Geometry: final body of the model. Coordinates: model frame, mm. A direction names the side the tool comes from. Coordinates: 2 decimals unless noted, no trailing zeros. Write each loop counter-clockwise with the first axis right and the second up, starting at its lowest first coordinate (ties: lowest second). Pieces come first, ordered by that corner, then holes.
Autodesk Inventor part; units mm, degrees
ref_plane "YZ Plane" through (0, 0, 0) normal (1, 0, 0) x (0, 1, 0)
ref_plane "XZ Plane" through (0, 0, 0) normal (0, 1, 0) x (-1, 0, 0)
ref_plane "XY Plane" through (0, 0, 0) normal (0, 0, 1) x (1, 0, 0)
sketch "Szkic1" plane through (0, 0, 0) normal (0, 0, 1) x (1, 0, 0)
  circle A0 centre (0, 0) radius 90
  circle A1 centre (0, 0) radius 90
  circle A2 centre (0, 0) radius 95
  point P0 (0, 0)
  dimension "d0" = 190
extrude "Wyciągnięcie proste1" add sketch "Szkic1" against normal blind 10
ref_plane "Płaszczyzna konstrukcyjna1" through (0, 0, 0) normal (0, 0, 1) x (1, 0, 0)
sketch "Szkic2" plane through (0, 0, 0) normal (0, 0, 1) x (1, 0, 0)
  circle A0 centre (0, 0) radius 95
  circle A1 centre (0, 0) radius 20
  dimension "d3" = 40
extrude "Wyciągnięcie proste2" add sketch "Szkic2" along normal blind 10
fillet "Zaokrąglenie1" radius 10 1 edges at (-95, 0, 10)
chamfer "Faza1" distance 2 angle 45 1 edges at (-95, 0, -10)
chamfer "Faza2" distance 2 angle 45 2 edges at (-20, 0, 0) (-20, 0, 10)
properties part number "dekieltop" material "PCW, nieplastyfikowany"
Item 1: Section A-A, the plane x = 0. Output: boundary loops of the cut face in (y, z).
Derived:
outline: (-95, -8) - (-93, -10) - (-90, -10) - (-90, 0) - (-22, 0) - (-20, 2) - (-20, 8) - (-22, 10) - (-85, 10) arc R10 ccw to (-95, 0) - close; (20, 2) - (22, 0) - (90, 0) - (90, -10) - (93, -10) - (95, -8) - (95, 0) arc R10 ccw to (85, 10) - (22, 10) - (20, 8) - close
Item 2: Set-up query: faces 1 (the flat face through (19, -19, 0)), 2 (the flat face through (-49, 76, -10)). Return all of +Z, -Z, +X, -X, +Y, -Y with unobstructed straight access to the full face (end or side cutting, diameter ignored); none if empty.
Derived:
face 1: -Z
face 2: -Z, +X, -X, +Y, -Y
Item 3: Pin query (flat end, axial travel): pin 1 (1 mm diameter, centred on y = 51, z = -3.5, fed in from +X); pin 2 (3 mm diameter, centred on x = -35.5, z = -6.5, fed in from +Y); pin 3 (1.5 mm diameter, centred on y = -12.5, z = -1.5, fed in from -X); pin 4 (24 mm diameter, centred on x = 0, y = 0, fed in from +Z). Return the tip coordinate at first contact, or that it passes through.
Derived:
pin 1: stops at x = 80.47
pin 2: stops at y = 88.71
pin 3: stops at x = -94.27
pin 4: passes through
Item 4: Material intervals for probe 1 along Y at (x, z) = (0, -7); probe 2 along Z at (x, y) = (59.5, -7.5); probe 3 along X at (y, z) = (-4.5, 8), sorted ascending.
Derived:
probe 1: y = -95 to -90, 90 to 95
probe 2: z = 0 to 10
probe 3: x = -90.89 to -19.49, 19.49 to 90.89
Item 5: Pull-direction query (Y, two-part tool) for faces 3 (the conical face through (88.825, 27.972, -9.875)), 4 (the conical face through (-4.36, 19.65, 1.87)), 5 (the conical face through (-4.36, -19.65, 8.13)), 6 (the flat face through (18, -18, 10)); classes: released by +Y, released by -Y, zero draft, split by the parting line, or undercut.
Derived:
face 3: split by the parting line
face 4: undercut
face 5: undercut
face 6: zero draft
